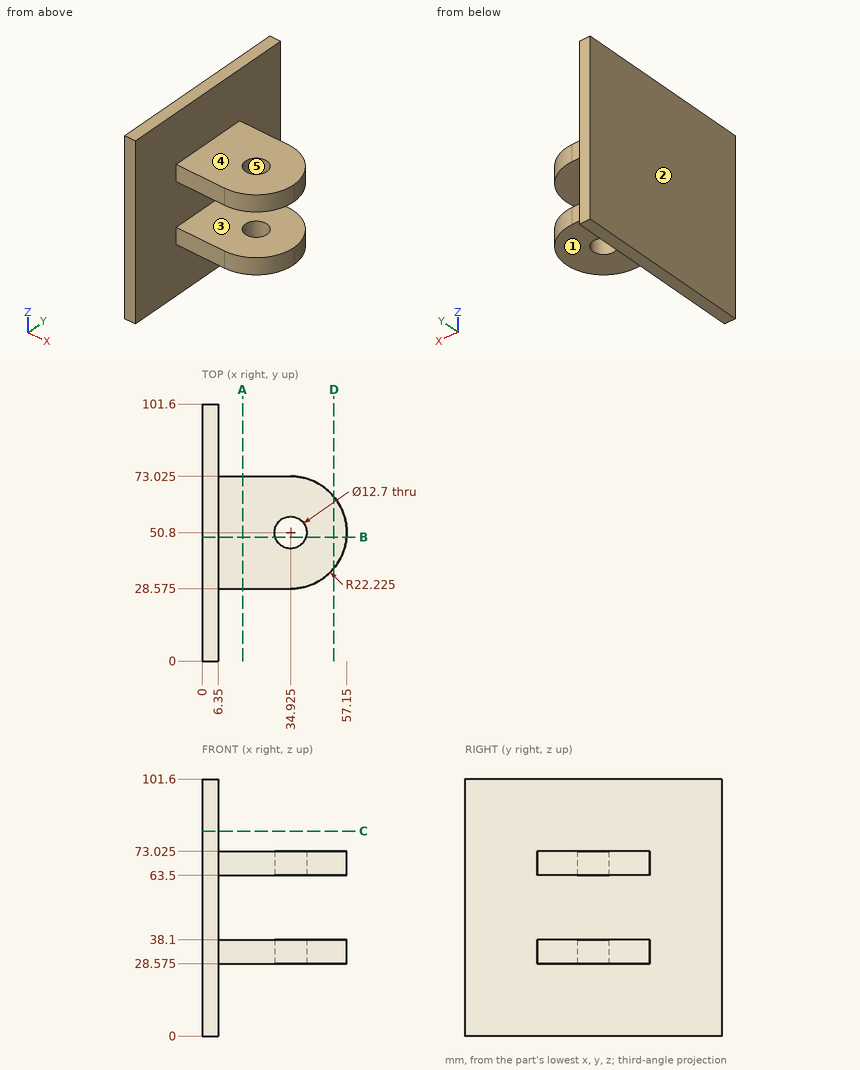
Job drawing, mm, ordinate dimensions from the low corner. One solid piece. A direction names the side the tool comes from. Give positions to 0.01 mm unless a question says otherwise; leave off trailing zeros. Write each loop counter-clockwise with the first axis right and the second up, starting at its lowest first coordinate (ties: lowest second). Pieces come first, ordered by that corner, then holes. Notation, with made-up numbers: M 38,22 L 92,22 A25 ccw 92,52 Z; hole C 2,-39 d8. An arc over 180 degrees is marked long. Put each result on its own line as item: value. Start each with the question number.
(1) Probe L1, parallel to Z at x = 16.5, y = 66 (3 decimals); L2, parallel to X at y = 97, z = 52.5; L3, parallel to X at y = 50, z = 65. List the from-to ranges inside material, lowest first.
(2) Band-saw the part on D-D, the plane x = 52. Write the cut outline in (y, z) (3 decimals), and give its area (3 significant figures).
(3) Band-saw the part on C-C, the plane z = 81. Write the cut outline in (x, y).
(4) Which spindle directions (+Z, -Z, +X, -X, +Y, -Y) get a long thin tool onto all of the face, cutting with end or side? Do the marked faces 1, 2 and 3. Say none if no direction does.
(5) Mould opens along Y. For the marked faces 4 and 5 say: +Y half, -Y half, draft (parallel to the pull), parting line (faces both ways), or undercut.
(6) Band-saw the part on B-B, the plane y = 49. Write the cut outline in (x, z) (3 decimals), and give its area (3 significant figures).
(7) Flat gauge pins, fed straight in: pin 1 Ø10 at (y, z) = (85, 54.5) entering from +X; pin 2 Ø13.5 at (x, y) = (23.5, 59.5) entering from -Z (3 decimals); pin 3 Ø7.5 at (x, y) = (34.925, 50.8) entering from -Z; pin 4 Ø22 at (x, y) = (36.5, 59.5) entering from +Z (3 decimals). Where does each tip first touch, or does it go through?
(8) Band-saw the part on A-A, the plane x = 16. Write the cut outline in (y, z) (3 decimals).
Response values:
1. L1: z = 28.575 to 38.1, 63.5 to 73.025
1. L2: x = 0 to 6.35
1. L3: x = 0 to 28.63, 41.22 to 57.14
2. outline: M 36.573,28.575 L 65.027,28.575 L 65.027,38.1 L 36.573,38.1 Z; M 36.573,63.5 L 65.027,63.5 L 65.027,73.025 L 36.573,73.025 Z
2. area: 542 mm2
3. outline: M 0,0 L 6.35,0 L 6.35,101.6 L 0,101.6 Z
4. face 1: -Z, +X, +Y, -Y
4. face 2: +Z, -Z, -X, +Y, -Y
4. face 3: +X, +Y, -Y
5. face 4: draft
5. face 5: undercut
6. outline: M 0,0 L 6.35,0 L 6.35,28.575 L 28.835,28.575 L 28.835,38.1 L 6.35,38.1 L 6.35,63.5 L 28.835,63.5 L 28.835,73.025 L 6.35,73.025 L 6.35,101.6 L 0,101.6 Z; M 41.015,28.575 L 57.077,28.575 L 57.077,38.1 L 41.015,38.1 Z; M 41.015,63.5 L 57.077,63.5 L 57.077,73.025 L 41.015,73.025 Z
6. area: 1,380 mm2
7. pin 1: stops at x = 6.35
7. pin 2: stops at z = 28.575
7. pin 3: passes through
7. pin 4: stops at z = 73.025
8. outline: M 28.575,28.575 L 73.025,28.575 L 73.025,38.1 L 28.575,38.1 Z; M 28.575,63.5 L 73.025,63.5 L 73.025,73.025 L 28.575,73.025 Z
